from build123d import *

# Parameters (mm, degrees)
BOSS_EXTRUDE2_DEPTH = 38.1
SKETCH8_R           = 5.715
BOSS_EXTRUDE3_DEPTH = 10.795
SKETCH9_W           = 5.715
SKETCH9_H           = 11.43
BOSS_EXTRUDE4_DEPTH = 10.795
SKETCH10_R          = 3.175
CUT_EXTRUDE1_DEPTH  = 10.795


with BuildPart() as part:
    # Sketch1 → Boss-Extrude2 (new body)
    with BuildSketch(Plane.XY):
        with BuildLine():
            Line((-21.59, 0), (-19.05, 0))
            ThreePointArc((-19.05, 0), (0, 19.05), (19.05, 0))
            Line((19.05, 0), (21.59, 0))
            ThreePointArc((21.59, 0), (0, 21.59), (-21.59, 0))
        make_face()
    extrude(amount=BOSS_EXTRUDE2_DEPTH)

    # Sketch8 → Boss-Extrude3 (add)
    with BuildSketch(Plane(origin=(0, 0, 0), x_dir=(1, 0, 0), z_dir=(0, 1, 0))):
        with Locations(Location((-24.765, -8.255, 0), (0, 0, 56.251011404))):
            Circle(SKETCH8_R)
        with Locations(Location((-24.765, -29.845, 0), (0, 0, 56.251011404))):
            Circle(SKETCH8_R)
    boss_extrude3 = extrude(amount=BOSS_EXTRUDE3_DEPTH)

    # Sketch9 → Boss-Extrude4 (add)
    with BuildSketch(Plane(origin=(0, 0, 0), x_dir=(1, 0, 0), z_dir=(0, 1, 0))):
        with Locations((-21.9075, -29.845)):
            Rectangle(SKETCH9_W, SKETCH9_H)
        with Locations((-21.9075, -8.255)):
            Rectangle(SKETCH9_W, SKETCH9_H)
    boss_extrude4 = extrude(amount=BOSS_EXTRUDE4_DEPTH)

    # Sketch10 → Cut-Extrude1 (cut)
    with BuildSketch(Plane(origin=(0, 10.795, 0), x_dir=(1, 0, 0), z_dir=(0, 1, 0))):
        with Locations(Location((-24.765, -29.845, 0), (0, 0, 270))):
            Circle(SKETCH10_R)
        with Locations(Location((-24.765, -8.255, 0), (0, 0, 270))):
            Circle(SKETCH10_R)
    cut_extrude1 = extrude(amount=-CUT_EXTRUDE1_DEPTH, mode=Mode.SUBTRACT)

    # Mirror1: Boss-Extrude3, Boss-Extrude4, Cut-Extrude1 across plane
    add(boss_extrude3.mirror(Plane(origin=(0, 0, 0), x_dir=(0, 0, 1), z_dir=(1, 0, 0))))
    add(boss_extrude4.mirror(Plane(origin=(0, 0, 0), x_dir=(0, 0, 1), z_dir=(1, 0, 0))))
    add(cut_extrude1.mirror(Plane(origin=(0, 0, 0), x_dir=(0, 0, 1), z_dir=(1, 0, 0))), mode=Mode.SUBTRACT)


solid = part.part
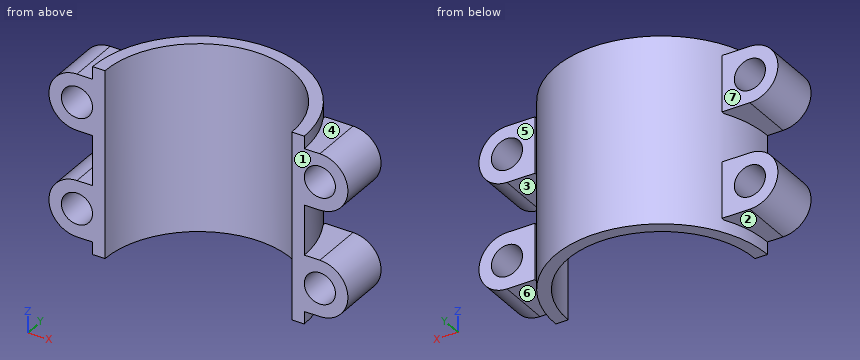
Read the model definition and answer for the solid it produces. Units are mm, in the model's axes. Face numbers are marked on the shaded views. A direction names the side the tool comes from. Give positions to 0.01 mm unless a question says otherwise; leave off trailing zeros. Write each loop counter-clockwise with the first axis right and the second up, starting at its lowest first coordinate (ties: lowest second). Pieces come first, ordered by that corner, then holes. Notation, with made-up numbers: (7.25, 28) - (52.25, 28) arc R27 ccw to (52.25, 55) - close; hole circle Ø4 at (39.5, 40). An arc over 180 degrees is marked (long way). Use CSV: the item, a comma, the result in double quotes. Start each with the question number.
(1) Given P1, Ø1.5, axis at x = 21, z = 24.5, coming from the +Y side (3 decimals); P2, Ø0.7, axis at y = 10.5, z = 6.5, coming from the +X side; P3, Ø10, axis at x = 21, z = 29.5, coming from the +Y side, each flat-ended and moving along its own axis, determine where each tip first touches the part or whether it passes through.
(2) Consider line 1 along Z through (x, y) = (-24, 9.5); line 2 along Z through (x, y) = (-21, 7.5); line 3 along X through (y, z) = (10.75, 26). Determine where each line is inside the solid, lowest interval first.
(3) Determine the mould class of the marked faces 1, 2 and 3 for opening direction Z: +Z half, -Z half, draft (parallel to the pull), parting line (faces both ways), or undercut.
(4) Find section C-C (y = 15.75). Give the vertices of the cut face in (x, z).
(5) Find section A-A (y = 7.5). Count the separate pieces of the cut face and the enclosed holes in it, plus the area to 4 significant figures.
(6) Find section D-D (x = 0). Give the vertices of the cut face in (y, z), plus the area to 3 significant figures.
(7) Find section B-B (z = 31). Give the vertices of the cut face in (x, y) (3 decimals), plus the area to 3 significant figures.
(8) For the marked faces 4, 5, 6 and 7, determine the directions among +Z, -Z, +X, -X, +Y, -Y from which every point of the face is accessible in a straight line to the end or side of a thin tool.
Findings below:
1,P1,"y = 10.795"
1,P2,"x = 30.3"
1,P3,"y = 14.5"
2,line 1,"2.54 to 5.17, 11.34 to 13.97, 24.13 to 26.76, 32.93 to 35.56"
2,line 2,"2.54 to 13.97, 24.13 to 35.56"
2,line 3,"-28.99 to -19.05, -18.72 to -15.73, 15.73 to 18.72, 19.05 to 28.99"
3,face 1,"draft"
3,face 2,"-Z half"
3,face 3,"undercut"
4,outline,"(-14.77, 0) - (-10.72, 0) - (-10.72, 38.1) - (-14.77, 38.1) - close; (10.72, 0) - (14.77, 0) - (14.77, 38.1) - (10.72, 38.1) - close"
5,separate pieces,"2"
5,enclosed holes,"4"
5,area,"493.5 mm2"
6,outline,"(19.05, 0) - (21.59, 0) - (21.59, 38.1) - (19.05, 38.1) - close"
6,area,"96.8 mm2"
7,outline,"(-30.362, 0) - (-27.722, 0) - (-27.722, 10.795) - (-30.362, 10.795) - close; (-21.808, 0) - (-19.05, 0) arc R19.05 cw to (19.05, 0) - (21.808, 0) - (21.808, 10.795) - (19.05, 10.795) - (19.05, 10.16) arc R21.59 ccw to (-19.05, 10.16) - (-19.05, 10.795) - (-21.808, 10.795) - close; (27.722, 0) - (30.362, 0) - (30.362, 10.795) - (27.722, 10.795) - close"
7,area,"244 mm2"
8,face 4,"+Z, +X, +Y"
8,face 5,"+Z, -Z, +X, +Y"
8,face 6,"-Z, +X, +Y"
8,face 7,"+Z, -Z, -X, +Y"
